Design review of the part built by this model. Coordinates are the model's own, in mm. Coordinates: 2 decimals unless noted, no trailing zeros.
```python
from build123d import *

# Parameters (mm, degrees)
BOX016_W     = 275
BOX016_H     = 275
BOX016_DEPTH = 59
SKETCH050_W  = 102
SKETCH050_H  = 102
SKETCH051_W  = 86
SKETCH051_H  = 86
BOX017_W     = 275
BOX017_H     = 275
BOX017_DEPTH = 46
SKETCH044_W  = 275
SKETCH044_H  = 275
SKETCH045_W  = 0.1
SKETCH045_H  = 0.1
SKETCH038_W  = 275
SKETCH038_H  = 275
SKETCH039_W  = 0.1
SKETCH039_H  = 0.1
BOX010_W     = 275
BOX010_H     = 275
BOX010_DEPTH = 70


with BuildPart() as layer0keep007:
    # Box016 → Box016 (new body)
    with BuildSketch(Plane.XY.offset(48)):
        with Locations((137.5, 137.5)):
            Rectangle(BOX016_W, BOX016_H)
    extrude(amount=BOX016_DEPTH)


with BuildPart() as obj1:
    # Sketch050 → Loft017 section 0
    with BuildSketch(Plane.XY.offset(107)):
        with Locations((137.5, 137.5)):
            Rectangle(SKETCH050_W, SKETCH050_H)
    # Sketch051 → Loft017 section 1
    with BuildSketch(Plane.XY.offset(117)):
        with Locations((137.5, 137.5)):
            Rectangle(SKETCH051_W, SKETCH051_H)
    loft()

    # Fusion021: union layer0Keep007
    add(layer0keep007.part)


with BuildPart() as obj1_1:
    # Fusion021 placement: moved
    add(obj1.part.moved(Location((0, 0, 1))))


with BuildPart() as layer2cut:
    # Box017 → Box017 (new body)
    with BuildSketch(Plane.XY.offset(123)):
        with Locations((137.5, 137.5)):
            Rectangle(BOX017_W, BOX017_H)
    extrude(amount=BOX017_DEPTH)


with BuildPart() as fusion022:
    # Sketch044 → Loft014 section 0
    with BuildSketch(Plane.XY):
        with Locations((137.5, 137.5)):
            Rectangle(SKETCH044_W, SKETCH044_H)
    # Sketch045 → Loft014 section 1
    with BuildSketch(Plane.XY.offset(175.1)):
        with Locations((137.5, 137.5)):
            Rectangle(SKETCH045_W, SKETCH045_H)
    loft()


with BuildPart() as fusion022_1:
    # Loft014 placement: moved
    add(fusion022.part.moved(Location((0, 0, -6))))

    # Common011: intersect layer2Cut
    add(layer2cut.part, mode=Mode.INTERSECT)

    # Fusion022: union obj1
    add(obj1_1.part)


with BuildPart() as obj2:
    # Sketch038 → Loft011 section 0
    with BuildSketch(Plane.XY):
        with Locations((137.5, 137.5)):
            Rectangle(SKETCH038_W, SKETCH038_H)
    # Sketch039 → Loft011 section 1
    with BuildSketch(Plane.XY.offset(175.1)):
        with Locations((137.5, 137.5)):
            Rectangle(SKETCH039_W, SKETCH039_H)
    loft()


with BuildPart() as layer2:
    # Box010 → Box010 (new body)
    with BuildSketch(Plane.XY.offset(108)):
        with Locations((137.5, 137.5)):
            Rectangle(BOX010_W, BOX010_H)
    extrude(amount=BOX010_DEPTH)

    # Common010: intersect obj2
    add(obj2.part, mode=Mode.INTERSECT)

    # Cut004: cut Fusion022
    add(fusion022_1.part, mode=Mode.SUBTRACT)


solid = layer2.part
```
(1) Insertion check: pin 1 Ø12 at (x, y) = (150, 160) entering from +Z; pin 2 Ø1 at (x, y) = (179.5, 122.5) entering from +Z; pin 3 Ø21.5 at (x, y) = (138, 148.5) entering from +Z. Each pin has a flat end and moves straight along its axis. Give the tip position at first contact, or say it passes through.
(2) Wall thickness on line 1 (X direction, y = 107.5, z = 127); line 2 (Z direction, x = 135, y = 132.5): over which ranges is each line inside the solid? List them lowest first.
(3) Mouldability with a two-part tool opening along X and no side actions: class faces 1 (the flat face through (136, 138, 118)), 2 (the flat face through (114, 189, 108)) as +X half, -X half, draft (parallel to the pull), parting line (faces both ways), or undercut.
Results:
1. pin 1: stops at z = 154.14
1. pin 2: stops at z = 122.3
1. pin 3: stops at z = 174.84
2. line 1: x = 99.69 to 104.4, 170.6 to 175.31
2. line 2: z = 118 to 123, 162.79 to 168.79
3. face 1: undercut
3. face 2: draft
